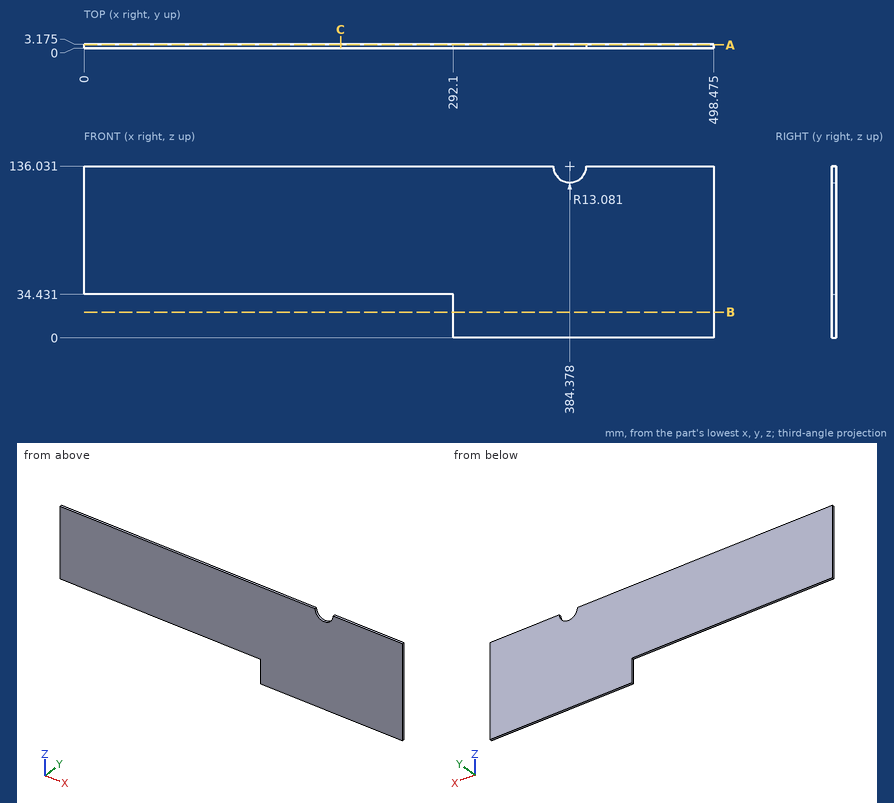
Job drawing, mm, ordinate dimensions from the low corner. One solid piece. Round coordinates to 2 decimals unless told otherwise and drop trailing zeros. Loops run counter-clockwise (first coordinate to the right, second up) from the corner with the lowest first, then second, coordinate; pieces in that order, holes last.
(1) Drop a flat-ended pin along its axis: pin 1 (1 mm diameter, centred on x = 154.5, y = 1.5, fed in from -Z). Give the stop position or say it passes through.
(2) Cut at A-A (y = 2.4). Give the cut face in (x, z) (1 decimal), plus the area to 3 significant figures.
(3) Wall check: line 1 along Z through (x, y) = (258, 1.4); line 2 along X through (y, z) = (1.45, 18.5) (1 decimal); line 3 along X through (y, z) = (0.25, 126) (1 decimal). Give the ranges that are in metal, low to high.
(4) Cut at C-C (x = 203). Give the cut face in (y, z) (1 decimal).
(5) Cut at B-B (z = 20.5). Give the cut face in (x, y) (1 decimal).
Findings below:
1. pin 1: stops at z = 34.43
2. outline: (0, 34.4) - (292.1, 34.4) - (292.1, 0) - (498.5, 0) - (498.5, 136) - (397.5, 136) arc R13.1 cw to (371.3, 136) - (0, 136) - close
2. area: 57,500 mm2
3. line 1: z = 34.43 to 136.03
3. line 2: x = 292.1 to 498.5
3. line 3: x = 0 to 376, 392.8 to 498.5
4. outline: (0, 34.4) - (3.2, 34.4) - (3.2, 136) - (0, 136) - close
5. outline: (292.1, 0) - (498.5, 0) - (498.5, 3.2) - (292.1, 3.2) - close
